Here's how the part is built. I have some questions about the finished solid (model axes, mm). Face numbers are marked on the shaded views. A direction names the side the tool comes from. Give positions to 0.01 mm unless a question says otherwise; leave off trailing zeros. Order: outer loops, then holes, each group sorted by start corner. A loop starts at its lowest first (then second) coordinate and runs counter-clockwise, first axis right, second up.
from build123d import *

# Parameters (mm, degrees)
SKETCH2_R           = 14
BOSS_EXTRUDE1_DEPTH = 12
SKETCH3_R           = 1.75
CUT_EXTRUDE1_DEPTH  = 13
SKETCH4_R           = 4.75
CUT_EXTRUDE2_DEPTH  = 4


with BuildPart() as part:
    # Sketch2 → Boss-Extrude1 (new body)
    with BuildSketch(Plane(origin=(0, 0, 12), x_dir=(-1, 0, 0), z_dir=(0, 0, -1))):
        Circle(SKETCH2_R)
    extrude(amount=BOSS_EXTRUDE1_DEPTH)

    # Sketch3 → Cut-Extrude1 (cut, through all)
    with BuildSketch(Plane.XY.offset(12)):
        with Locations((-6.479247663, 4.692477993)):
            Circle(SKETCH3_R)
        with Locations((5.572317617, 7.6941066)):
            Circle(SKETCH3_R)
        with Locations((6.479247663, -4.692477993)):
            Circle(SKETCH3_R)
        with Locations((-5.572317617, -7.6941066)):
            Circle(SKETCH3_R)
    extrude(amount=-CUT_EXTRUDE1_DEPTH, mode=Mode.SUBTRACT)

    # Sketch4 → Cut-Extrude2 (cut)
    with BuildSketch(Plane.XY.offset(12)):
        Circle(SKETCH4_R)
    extrude(amount=-CUT_EXTRUDE2_DEPTH, mode=Mode.SUBTRACT)


solid = part.part
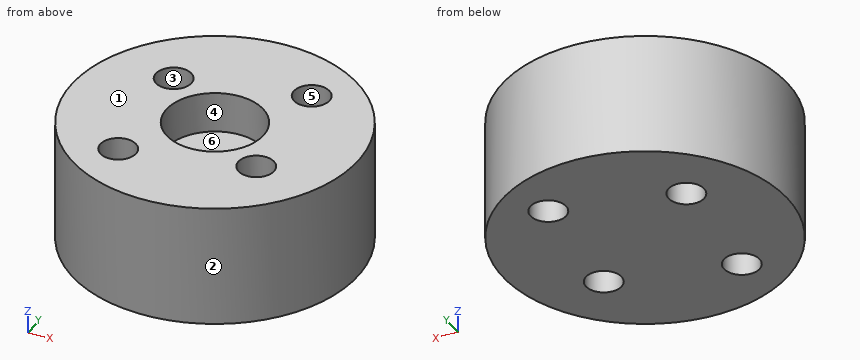
Q1. I need wall thicknesses on L1, parallel to Y at x = 0, z = 9.6; L2, parallel to X at y = 3.5, z = 2.75; L3, parallel to X at y = -6.75, z = 1.5. Which ranges of each line are inside material? Lowest first, please.
Filled sheet:
L1: y = -14 to -4.75, 4.75 to 14
L2: x = -13.56 to -7.76, -5.2 to 13.56
L3: x = -12.27 to -7.05, -4.1 to 12.27
Q2. If we section it at D-D on z = 8.5: List the corners of the cut face in (x, y) for me, plus the area to 3 significant figures.
Filled sheet:
outline: circle Ø28 at (0, 0); hole circle Ø3.5 at (-6.48, 4.69); hole circle Ø3.5 at (-5.57, -7.69); hole circle Ø9.5 at (0, 0); hole circle Ø3.5 at (5.57, 7.69); hole circle Ø3.5 at (6.48, -4.69)
area: 506 mm2
Q3. I'm going to push flat-ended pins straight in: P1, Ø1, axis at x = -4, z = 7.5, coming from the +Y side; P2, Ø1, axis at y = 10, z = 5, coming from the -X side; P3, Ø3, axis at x = 7.5, z = 4, coming from the +Y side. Where does each tip first touch, or does it pass through?
Filled sheet:
P1: stops at y = 13.56
P2: stops at x = -10.28
P3: stops at y = 12.65
Q4. If we section it at A-A on x = 0: List the corners of the cut face in (y, z) for me, plus the area to 3 significant figures.
Filled sheet:
outline: (-14, 0) - (14, 0) - (14, 12) - (4.75, 12) - (4.75, 8) - (-4.75, 8) - (-4.75, 12) - (-14, 12) - close
area: 298 mm2
Q5. For the marked faces 5 and 6, which set-ups out of +Z, -Z, +X, -X, +Y, -Y let a thin tool reach every point of the face, with its end or its side?
Filled sheet:
face 5: +Z, -Z
face 6: +Z
Q6. If we section it at C-C on z = 2.5: List the corners of the cut face in (x, y) for me, plus the area to 3 significant figures.
Filled sheet:
outline: circle Ø28 at (0, 0); hole circle Ø3.5 at (-6.48, 4.69); hole circle Ø3.5 at (-5.57, -7.69); hole circle Ø3.5 at (5.57, 7.69); hole circle Ø3.5 at (6.48, -4.69)
area: 577 mm2
Q7. Thinking about a two-plate mould opening in X: for the marked faces 1, 2, 3 and 4, which applies, released by +X, released by -X, zero draft, split by the parting line, or undercut?
Filled sheet:
face 1: zero draft
face 2: split by the parting line
face 3: undercut
face 4: undercut
